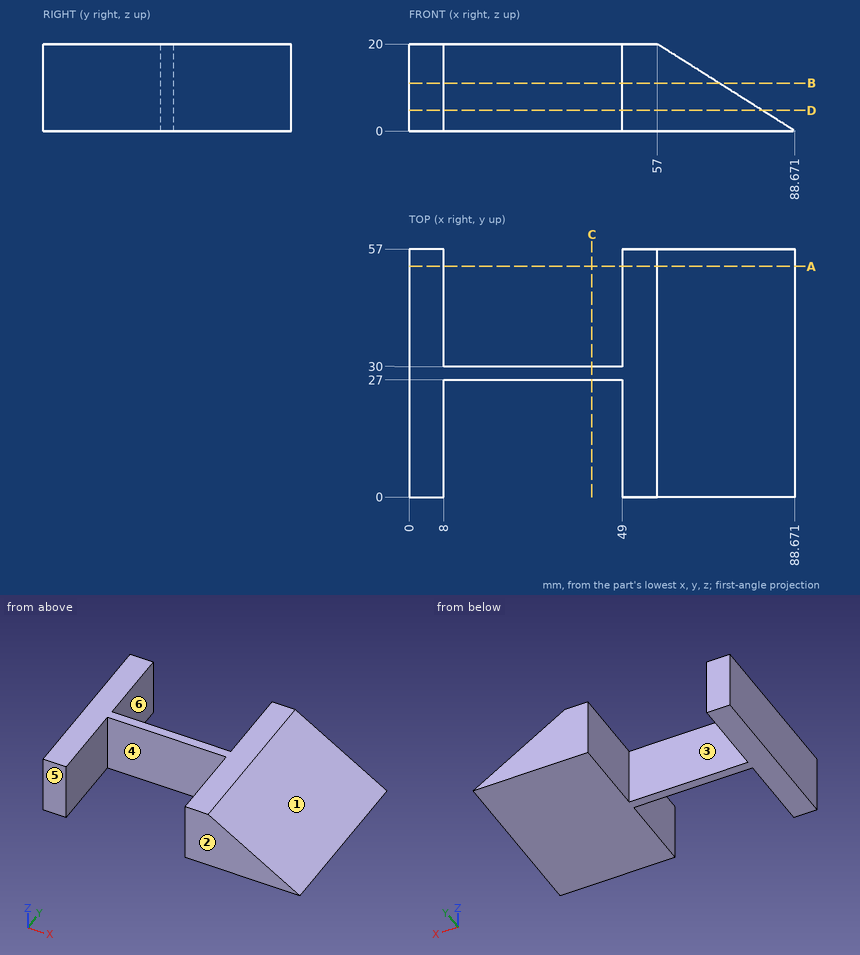
Drawing for the job (mm, zero at the part's lowest x, y, z). A direction names the side the tool comes from. Give positions to 0.01 mm unless a question says otherwise; leave off trailing zeros. Order: outer loops, then holes, each group sorted by start corner. A loop starts at its lowest first (then second) coordinate and runs counter-clockwise, first axis right, second up. Notation, with made-up numbers: M -31.5,2 L 8.5,2 A27 ccw 8.5,35 Z; hole C -32.5,86.5 d5. An arc over 180 degrees is marked long. Put each result on its own line as item: value. Start each with the question number.
(1) Mould opens along X. For the marked faces 1, 2 and 3 say: +X half, -X half, draft (parallel to the pull), parting line (faces both ways), or undercut.
(2) Flat gauge pins, fed straight in: pin 1 Ø4 at (x, z) = (37.5, 6) entering from -Y; pin 2 Ø1 at (x, y) = (66, 37) entering from +Z. Where does each tip first touch, or does it go through?
(3) Saw through at C-C, the plane x = 42. Write the cut outline in (y, z).
(4) Drill centre lines: line 1 along Y through (x, z) = (19, 6.25); line 2 along X through (y, z) = (53, 5.5); line 3 along X through (y, z) = (37, 9). Where is each one in solid material? Low to high.
(5) Saw through at B-B, the plane z = 11. Write the cut outline in (x, y).
(6) Saw through at D-D, the plane z = 4.75. Write the cut outline in (x, y).
(7) Which spindle directions (+Z, -Z, +X, -X, +Y, -Y) get a long thin tool onto all of the face, cutting with end or side? Do the marked faces 4, 5 and 6. Say none if no direction does.
(8) Saw through at A-A, the plane y = 53. Write the cut outline in (x, z).
Check result:
1. face 1: +X half
1. face 2: draft
1. face 3: undercut
2. pin 1: stops at y = 27
2. pin 2: stops at z = 14.63
3. outline: M 27,0 L 30,0 L 30,20 L 27,20 Z
4. line 1: y = 27 to 30
4. line 2: x = 0 to 8, 49 to 79.96
4. line 3: x = 0 to 8, 49 to 74.42
5. outline: M 0,0 L 8,0 L 8,27 L 49,27 L 49,0 L 71.25,0 L 71.25,57 L 49,57 L 49,30 L 8,30 L 8,57 L 0,57 Z
6. outline: M 0,0 L 8,0 L 8,27 L 49,27 L 49,0 L 81.15,0 L 81.15,57 L 49,57 L 49,30 L 8,30 L 8,57 L 0,57 Z
7. face 4: +Z, -Z, -Y
7. face 5: +Z, -Z, +X, -X, -Y
7. face 6: +Z, -Z, +Y
8. outline: M 0,0 L 8,0 L 8,20 L 0,20 Z; M 49,0 L 88.67,0 L 57,20 L 49,20 Z
